Autodesk Inventor part; units mm, degrees
ref_plane "YZ Plane" through (0, 0, 0) normal (1, 0, 0) x (0, 1, 0)
ref_plane "XZ Plane" through (0, 0, 0) normal (0, 1, 0) x (-1, 0, 0)
ref_plane "XY Plane" through (0, 0, 0) normal (0, 0, 1) x (1, 0, 0)
sketch "Sketch1" plane through (0, 0, 0) normal (0, 1, 0) x (-1, 0, 0)
  line L0 (60, 8) -> (-60, 8)
  line L1 (-60, 8) -> (-60, -8)
  line L2 (-60, -8) -> (60, -8)
  line L3 (60, -8) -> (60, 8)
  line L4 (60, 8) -> (-60, -8) construction
  line L5 (-60, 8) -> (60, -8) construction
  point P0 (0, 0)
  dimension "d0" = 16
  dimension "d1" = 120
extrude "Extrusion1" add sketch "Sketch1" along normal blind 10
hole "Hole1" at (0, 10, 0) direction (0, -1, 0) diameter 7.142 depth 25.4 counterbore diameter 11.113 counterbore depth 6.35
sketch "Sketch2" plane through (0, 10, 0) normal (0, 1, 0) x (1, 0, 0)
  circle A0 centre (15, 0) radius 2.75
  circle A1 centre (45, 0) radius 2.75
  circle A2 centre (-15, 0) radius 2.75
  circle A3 centre (-45, 0) radius 2.75
  point P0 (0, 0)
  dimension "d15" = 5.5
  dimension "d16" = 15
  dimension "d17" = 30
  dimension "d18" = 5.5
  dimension "d19" = 15
  dimension "d20" = 5.5
  dimension "d21" = 30
  dimension "d22" = 5.5
extrude "Extrusion2" cut sketch "Sketch2" against normal up to next
properties part number "flowmeter_mount"
Part model, mm, in its own coordinate system. A direction names the side the tool comes from. Round coordinates to 2 decimals unless told otherwise and drop trailing zeros. Loops run counter-clockwise (first coordinate to the right, second up) from the corner with the lowest first, then second, coordinate; pieces in that order, holes last. Notation, with made-up numbers: (-17, 8.25) -> (-3, 8.25) arc R21 cw to (-3, 39.25) -> close; hole circle Ø7 at (34.5, 11). An arc over 180 degrees is marked (long way). Use one line per item in the form item = value. Start each with the question number.
Item 1: Drill centre lines: line 1 along X through (y, z) = (7.5, 0); line 2 along Z through (x, y) = (0, 7); line 3 along X through (y, z) = (2.1, 0). Where is each one in solid material? Low to high.
Item 2: Drop a flat-ended pin along its axis: pin 1 Ø3.5 at (x, z) = (0.5, 1) entering from +Y. Give the stop position or say it passes through.
Item 3: Band-saw the part on B-B (z = 0). List the corners of the cut face in (x, y), plus the area to 3 significant figures.
Item 4: Two-plate mould, pull along Z, no slides. Class faces 1 (the cylindrical face through (12.253, 5.07, -0.121)), 2 (the flat face through (-60, 5, 0)), 3 (the flat face through (-1, 5, 8)): released by +Z, released by -Z, zero draft, split by the parting line, or undercut.
Item 5: Band-saw the part on C-C (y = 8.25). List the corners of the cut face in (x, z), plus the area to 3 significant figures.
Item 6: Band-saw the part on D-D (x = 15). List the corners of the cut face in (y, z), plus the area to 3 significant figures.
Item 7: Band-saw the part on A-A (x = 0). List the corners of the cut face in (y, z), plus the area to 3 significant figures.
Item 8: Tool access for faces 4 (the flat face through (60, 5, 0)), 5 (the flat face through (4, 3.65, 0)): list every direction of +Z, -Z, +X, -X, +Y, -Y with a clear straight run to the whole face (end or side of a thin tool).
Data:
q1.line_1 = -60 to -47.75, -42.25 to -17.75, -12.25 to -5.56, 5.56 to 12.25, 17.75 to 42.25, 47.75 to 60
q1.line_2 = -8 to -5.56, 5.56 to 8
q1.line_3 = -60 to -47.75, -42.25 to -17.75, -12.25 to -3.57, 3.57 to 12.25, 17.75 to 42.25, 47.75 to 60
q2.pin_1 = through
q3.outline = (-60, 0) -> (-47.75, 0) -> (-47.75, 10) -> (-60, 10) -> close; (-42.25, 0) -> (-17.75, 0) -> (-17.75, 10) -> (-42.25, 10) -> close; (-12.25, 0) -> (-3.57, 0) -> (-3.57, 3.65) -> (-5.56, 3.65) -> (-5.56, 10) -> (-12.25, 10) -> close; (3.57, 0) -> (12.25, 0) -> (12.25, 10) -> (5.56, 10) -> (5.56, 3.65) -> (3.57, 3.65) -> close; (17.75, 0) -> (42.25, 0) -> (42.25, 10) -> (17.75, 10) -> close; (47.75, 0) -> (60, 0) -> (60, 10) -> (47.75, 10) -> close
q3.area = 883 mm^2
q4.face_1 = undercut
q4.face_2 = zero draft
q4.face_3 = released by +Z
q5.outline = (-60, -8) -> (60, -8) -> (60, 8) -> (-60, 8) -> close; hole circle Ø5.5 at (-45, 0); hole circle Ø5.5 at (-15, 0); hole circle Ø11.11 at (0, 0); hole circle Ø5.5 at (15, 0); hole circle Ø5.5 at (45, 0)
q5.area = 1,730 mm^2
q6.outline = (0, -8) -> (10, -8) -> (10, -2.75) -> (0, -2.75) -> close; (0, 2.75) -> (10, 2.75) -> (10, 8) -> (0, 8) -> close
q6.area = 105 mm^2
q7.outline = (0, -8) -> (10, -8) -> (10, -5.56) -> (3.65, -5.56) -> (3.65, -3.57) -> (0, -3.57) -> close; (0, 3.57) -> (3.65, 3.57) -> (3.65, 5.56) -> (10, 5.56) -> (10, 8) -> (0, 8) -> close
q7.area = 63.4 mm^2
q8.face_4 = +Z, -Z, +X, +Y, -Y
q8.face_5 = +Y
